Source: CAD feature listing. Evaluate the final solid. Frame: model axes, mm. Face numbers are marked on the shaded views. Coordinates: 2 decimals unless noted, no trailing zeros. Order: outer loops, then holes, each group sorted by start corner. A loop starts at its lowest first (then second) coordinate and runs counter-clockwise, first axis right, second up. Notation, with made-up numbers: (9, 59.5) -> (49, 59.5) arc R24 cw to (49, 72.5) -> close; hole circle Ø3 at (22.25, -17). An arc over 180 degrees is marked (long way). Put each result on its own line as item: value.
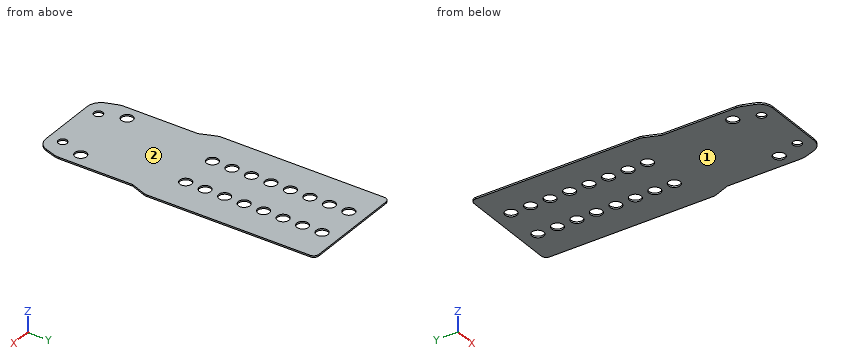
from build123d import *

# Parameters (mm, degrees)
BOSS_EXTRUDE1_DEPTH = 0.6096
SKETCH3_R           = 1.7
SKETCH3_R_2         = 2.25
CUT_EXTRUDE1_DEPTH  = 116.89918728
SKETCH5_R           = 2.25
CUT_EXTRUDE2_DEPTH  = 116.89918728
LPATTERN1_COUNT     = 7
LPATTERN1_PITCH     = 7.5
BOSS_EXTRUDE2_START = -0.6096
BOSS_EXTRUDE2_DEPTH = 0.6096


with BuildPart() as part:
    # Sketch2 → Boss-Extrude1 (new body)
    with BuildSketch(Plane.XY):
        with BuildLine():
            Line((34.883504, 3.686554855), (36.164103759, 7.513864099))
            ThreePointArc((36.164103759, 7.513864099), (36.415476383, 8.531517689), (36.5, 9.576344365))
            Line((36.5, 9.576344365), (36.5, 108))
            ThreePointArc((36.5, 108), (35.914213562, 109.414213562), (34.5, 110))
            Line((34.5, 110), (2, 110))
            ThreePointArc((2, 110), (0.585786438, 109.414213562), (0, 108))
            Line((0, 108), (0, 9.576344365))
            ThreePointArc((0, 9.576344365), (0.084523617, 8.531517689), (0.335896241, 7.513864099))
            Line((0.335896241, 7.513864099), (1.616496, 3.686554855))
            ThreePointArc((1.616496, 3.686554855), (3.582495544, 1.017500497), (6.737443738, 0))
            Line((6.737443738, 0), (29.762556262, 0))
            ThreePointArc((29.762556262, 0), (32.917504456, 1.017500497), (34.883504, 3.686554855))
        make_face()
    extrude(amount=BOSS_EXTRUDE1_DEPTH)

    # Sketch3 → Cut-Extrude1 (cut, through all)
    with BuildSketch(Plane.XY.offset(0.6096)):
        with Locations((8.25, 5.4)):
            Circle(SKETCH3_R)
        with Locations((5.25, 14.4)):
            Circle(SKETCH3_R_2)
        with Locations((10.75, 103.5)):
            Circle(SKETCH3_R_2)
        with Locations(Location((28.25, 5.4, 0), (0, 0, 180))):
            Circle(SKETCH3_R)
        with Locations(Location((31.25, 14.4, 0), (0, 0, 180))):
            Circle(SKETCH3_R_2)
        with Locations(Location((25.75, 103.5, 0), (0, 0, 180))):
            Circle(SKETCH3_R_2)
    extrude(amount=-CUT_EXTRUDE1_DEPTH, mode=Mode.SUBTRACT)

    # Sketch5 → Cut-Extrude2 (cut, through all)
    with BuildSketch(Plane.XY.offset(0.6096)):
        with Locations((10.75, 96)):
            Circle(SKETCH5_R)
        with Locations((25.75, 96)):
            Circle(SKETCH5_R)
    cut_extrude2 = extrude(amount=-CUT_EXTRUDE2_DEPTH, mode=Mode.SUBTRACT)

    # LPattern1: Cut-Extrude2 ×7
    with Locations(*[(0, -i * LPATTERN1_PITCH, 0) for i in range(1, LPATTERN1_COUNT)]):
        add(cut_extrude2, mode=Mode.SUBTRACT)

    # Sketch7 → Boss-Extrude2 (add)
    with BuildSketch(Plane.XY.offset(0.6096).offset(BOSS_EXTRUDE2_START)):
        with BuildLine():
            ThreePointArc((0, 108), (0.585786438, 109.414213562), (2, 110))
            Line((2, 110), (-0.5, 110))
            ThreePointArc((-0.5, 110), (-1.914213562, 109.414213562), (-2.5, 108))
            Line((-2.5, 108), (-2.5, 45.242710622))
            ThreePointArc((-2.5, 45.242710622), (-2.432780804, 44.512481103), (-2.233382425, 43.806794305))
            Line((-2.233382425, 43.806794305), (0, 38))
            Line((0, 38), (0, 108))
        make_face()
        with BuildLine():
            Line((36.5, 108), (36.5, 38))
            Line((36.5, 38), (38.733382425, 43.806794305))
            ThreePointArc((38.733382425, 43.806794305), (38.932780804, 44.512481103), (39, 45.242710622))
            Line((39, 45.242710622), (39, 108))
            ThreePointArc((39, 108), (38.414213562, 109.414213562), (37, 110))
            Line((37, 110), (34.5, 110))
            ThreePointArc((34.5, 110), (35.914213562, 109.414213562), (36.5, 108))
        make_face()
    extrude(amount=BOSS_EXTRUDE2_DEPTH)


solid = part.part
1. Cut plane A-A on y = 66. Output: boundary loops of the cut face in (x, z), plus the area to 3 significant figures.
Numbers:
outline: (-2.5, 0) -> (8.5, 0) -> (8.5, 0.61) -> (-2.5, 0.61) -> close; (13, 0) -> (23.5, 0) -> (23.5, 0.61) -> (13, 0.61) -> close; (28, 0) -> (39, 0) -> (39, 0.61) -> (28, 0.61) -> close
area: 19.8 mm2
2. Pull-direction query (Z, two-part tool) for the marked faces 1 and 2; classes: pulls with the +Z half, pulls with the -Z half, needs draft (parallel to the pull), parting line crosses it, or undercut.
Numbers:
face 1: pulls with the -Z half
face 2: pulls with the +Z half
3. Cut plane D-D on y = 22.5. Output: boundary loops of the cut face in (x, z).
Numbers:
outline: (0, 0) -> (36.5, 0) -> (36.5, 0.61) -> (0, 0.61) -> close
4. Ray query, line 1 along X through (y, z) = (64, 0.4); line 2 along X through (y, z) = (17, 0.35); line 3 along Y through (x, z) = (5.25, 0.4). Return the intervals inside material, ascending.
Numbers:
line 1: x = -2.5 to 9.72, 11.78 to 24.72, 26.78 to 39
line 2: x = 0 to 36.5
line 3: y = 0.21 to 12.15, 16.65 to 110
5. Cut plane B-B on x = 5.25. Output: boundary loops of the cut face in (y, z), plus the area to 3 significant figures.
Numbers:
outline: (0.21, 0) -> (12.15, 0) -> (12.15, 0.61) -> (0.21, 0.61) -> close; (16.65, 0) -> (110, 0) -> (110, 0.61) -> (16.65, 0.61) -> close
area: 64.2 mm2
6. Cut plane C-C on z = 0.15. Count the separate pieces of the cut face and the enclosed holes in it, plus the area to 3 significant figures.
Numbers:
separate pieces: 1
enclosed holes: 20
area: 4,020 mm2
7. First-contact query: pin 1 (4 mm diameter, centred on x = 25.75, y = 58.5, fed in from -Z) (3 decimals). Flat tip, straight axial feed; report the tip coordinate or a pass-through.
Numbers:
pin 1: passes through
